Read the model definition and answer for the solid it produces. Units are mm, in the model's axes. Coordinates: 2 decimals unless noted, no trailing zeros. Write each loop counter-clockwise with the first axis right and the second up, starting at its lowest first coordinate (ties: lowest second). Pieces come first, ordered by that corner, then holes.
Item 1: Section B-B (z = 7) is taken. Give the vertices of the cut face in (x, y), then the cut area to 3 significant figures.
Item 2: Section C-C (y = -79) is taken. Give the vertices of the cut face in (x, z).
Item 3: Section D-D (z = 0) is taken. Give the vertices of the cut face in (x, y).
Item 4: Section A-A (x = 0) is taken. Give the vertices of the cut face in (y, z).
Item 5: Straight lines are drawn through the part: probe 1 along Y at (x, z) = (7.5, 0); probe 2 along Y at (x, z) = (-4.25, 3.75); probe 3 along Z at (x, y) = (-0.25, -50). For each, find the intervals that lie inside material, in ascending order.
Item 6: Each of these flat-tipped pins is pushed along its axis until it touches: P1, Ø1.5, axis at y = -94.5, z = 8, coming from the -X side; P2, Ø2, axis at y = -11, z = 1, coming from the +X side; P3, Ø2, axis at y = -72.5, z = -0.5, coming from the -X side. Where does it stop, or does it pass through?
from build123d import *

# Parameters (mm, degrees)
F0_R     = 5
F1_DEPTH = 100


with BuildPart() as f1:
    # F0 (on Front) → F1 (new body)
    with BuildSketch(Plane.XZ):
        Circle(F0_R)
    extrude(amount=F1_DEPTH)

    # F2 (on Right) → F3 (revolve)
    with BuildSketch(Plane.YZ):
        with BuildLine():
            Line((0, -10), (0, 10))
            ThreePointArc((0, 10), (-5, 8.6602540378), (-8.6602540378, 5))
            ThreePointArc((-8.6602540378, 5), (-10, 0), (-8.6602540378, -5))
            ThreePointArc((-8.6602540378, -5), (-5, -8.6602540378), (0, -10))
        make_face()
    revolve(axis=Axis((0, 0, 0), (0, 0, -1)))

    # F2 (on Right) → F4 (revolve)
    with BuildSketch(Plane.YZ):
        with BuildLine():
            ThreePointArc((-91.3397459622, -5), (-90, 0), (-91.3397459622, 5))
            ThreePointArc((-91.3397459622, 5), (-95, 8.6602540378), (-100, 10))
            Line((-100, 10), (-100, -10))
            ThreePointArc((-100, -10), (-95, -8.6602540378), (-91.3397459622, -5))
        make_face()
    revolve(axis=Axis((0, -100, 0), (0, 0, -1)))


solid = f1.part
Established:
1. outline: circle Ø14.28 at (0, -100); circle Ø14.28 at (0, 0)
1. area: 320 mm2
2. outline: circle Ø10 at (0, 0)
3. outline: (-5, -91.34) arc R10 ccw (long way) to (5, -91.34) - (5, -8.66) arc R10 ccw (long way) to (-5, -8.66) - close
4. outline: (-91.34, -5) - (-8.66, -5) arc R10 ccw (long way) to (-8.66, 5) - (-91.34, 5) arc R10 ccw (long way) to start
5. probe 1: y = -106.61 to -93.39, -6.61 to 6.61
5. probe 2: y = -108.24 to -91.76, -8.24 to 8.24
5. probe 3: z = -4.99 to 4.99
6. P1: stops at x = -4.44
6. P2: stops at x = 5
6. P3: stops at x = -5
